Read the model definition and answer for the solid it produces. Units are mm, in the model's axes. A direction names the side the tool comes from. Give positions to 0.01 mm unless a question says otherwise; leave off trailing zeros. Write each loop counter-clockwise with the first axis right and the second up, starting at its lowest first coordinate (ties: lowest second). Pieces come first, ordered by that corner, then holes. Notation, with made-up numbers: (44, 73) -> (79, 73) arc R25 cw to (79, 97) -> close; hole circle Ø10 at (-8, 66). An arc over 180 degrees is marked (long way). Use a Markdown table: item, result.
from build123d import *

# Parameters (mm, degrees)
F0_W     = 6
F0_H     = 6
F1_DEPTH = 3.2
F2_R     = 1.75
F3_DEPTH = 2
F4_R     = 0.5
F5_DEPTH = 3


with BuildPart() as f1:
    # F0 (on Top) → F1 (new body)
    with BuildSketch(Plane.XY):
        Rectangle(F0_W, F0_H)
    extrude(amount=-F1_DEPTH)

    # F2 (on face) → F3 (join)
    with BuildSketch(Plane.XY):
        Circle(F2_R)
    extrude(amount=F3_DEPTH)

    # F4 (on face) → F5 (join)
    with BuildSketch(Plane(origin=(0, 0, -3.2), x_dir=(1, 0, 0), z_dir=(0, 0, -1))):
        with Locations((-3, 2.4)):
            Circle(F4_R)
        with Locations((3, 2.4)):
            Circle(F4_R)
        with Locations((-3, -2.4)):
            Circle(F4_R)
        with Locations((3, -2.4)):
            Circle(F4_R)
    extrude(amount=F5_DEPTH)


solid = f1.part
Item 1: Each of these flat-tipped pins is pushed along its axis until it touches: P1, Ø3, axis at x = -1, y = 0, coming from the -Z side; P2, Ø1.6, axis at y = 0, z = -1, coming from the +X side; P3, Ø0.6, axis at x = 3, y = -2.5, coming from the +Z side. Where does it stop, or does it pass through?
Return value:
| item | result |
|---|---|
| P1 | z = -3.2 |
| P2 | x = 3 |
| P3 | z = 0 |
Item 2: A cutting plane is placed at D-D (y = 1.05). Give the vertices of the cut face in (x, z), then the cut area to 3 significant figures.
Return value:
| item | result |
|---|---|
| outline | (-3, -3.2) -> (3, -3.2) -> (3, 0) -> (1.4, 0) -> (1.4, 2) -> (-1.4, 2) -> (-1.4, 0) -> (-3, 0) -> close |
| area | 24.8 mm^2 |
Item 3: Straight lines are drawn through the part: line 1 along X through (y, z) = (-2.25, -2); line 2 along Z through (x, y) = (0.5, 1.25); line 3 along Z through (x, y) = (-2.5, 1.8). For each, find the intervals that lie inside material, in ascending order. Write a range as [from, to].
Return value:
| item | result |
|---|---|
| line 1 | [-3, 3] |
| line 2 | [-3.2, 2] |
| line 3 | [-3.2, 0] |
Item 4: A cutting plane is placed at A-A (y = 2.4). Give the vertices of the cut face in (x, z).
Return value:
| item | result |
|---|---|
| outline | (-3.5, -6.2) -> (-2.5, -6.2) -> (-2.5, -3.2) -> (2.5, -3.2) -> (2.5, -6.2) -> (3.5, -6.2) -> (3.5, -3.2) -> (3, -3.2) -> (3, 0) -> (-3, 0) -> (-3, -3.2) -> (-3.5, -3.2) -> close |
Item 5: A cutting plane is placed at C-C (x = 0). Give the vertices of the cut face in (y, z).
Return value:
| item | result |
|---|---|
| outline | (-3, -3.2) -> (3, -3.2) -> (3, 0) -> (1.75, 0) -> (1.75, 2) -> (-1.75, 2) -> (-1.75, 0) -> (-3, 0) -> close |
Item 6: A tool of negligible diameter and unlimited length cuts with its end or side. For faces 1 (the face through (0, 0, -3.2)), 2 (the face through (-3, 0, -2)), 3 (the face through (3, 0, -2)), 4 (the face through (1.3, 1.4, 0)), from which of +Z, -Z, +X, -X, +Y, -Y can it reach the whole face along a straight path? Write none if from no direction.
Return value:
| item | result |
|---|---|
| face 1 | -Z |
| face 2 | +Z, -X, +Y, -Y |
| face 3 | +Z, +X, +Y, -Y |
| face 4 | +Z |
Item 7: A cutting plane is placed at B-B (z = -4). Give the vertices of the cut face in (x, y).
Return value:
| item | result |
|---|---|
| outline | circle Ø1 at (-3, -2.4); circle Ø1 at (-3, 2.4); circle Ø1 at (3, -2.4); circle Ø1 at (3, 2.4) |
Item 8: For a pull along Y with two mould halves and no side action, classify faces 5 (the face through (2.6, -2.7, -4.7)), 6 (the face through (0, 3, -2)), 7 (the face through (3, -2.4, -6.2)) as +Y half, -Y half, draft (parallel to the pull), parting line (faces both ways), or undercut.
Return value:
| item | result |
|---|---|
| face 5 | undercut |
| face 6 | +Y half |
| face 7 | draft |
